The drawing under review shows one solid part. Ordinate dimensions are in mm from its lowest x, y, z. A direction names the side the tool comes from. Coordinates: 2 decimals unless noted, no trailing zeros. Order: outer loops, then holes, each group sorted by start corner. A loop starts at its lowest first (then second) coordinate and runs counter-clockwise, first axis right, second up.
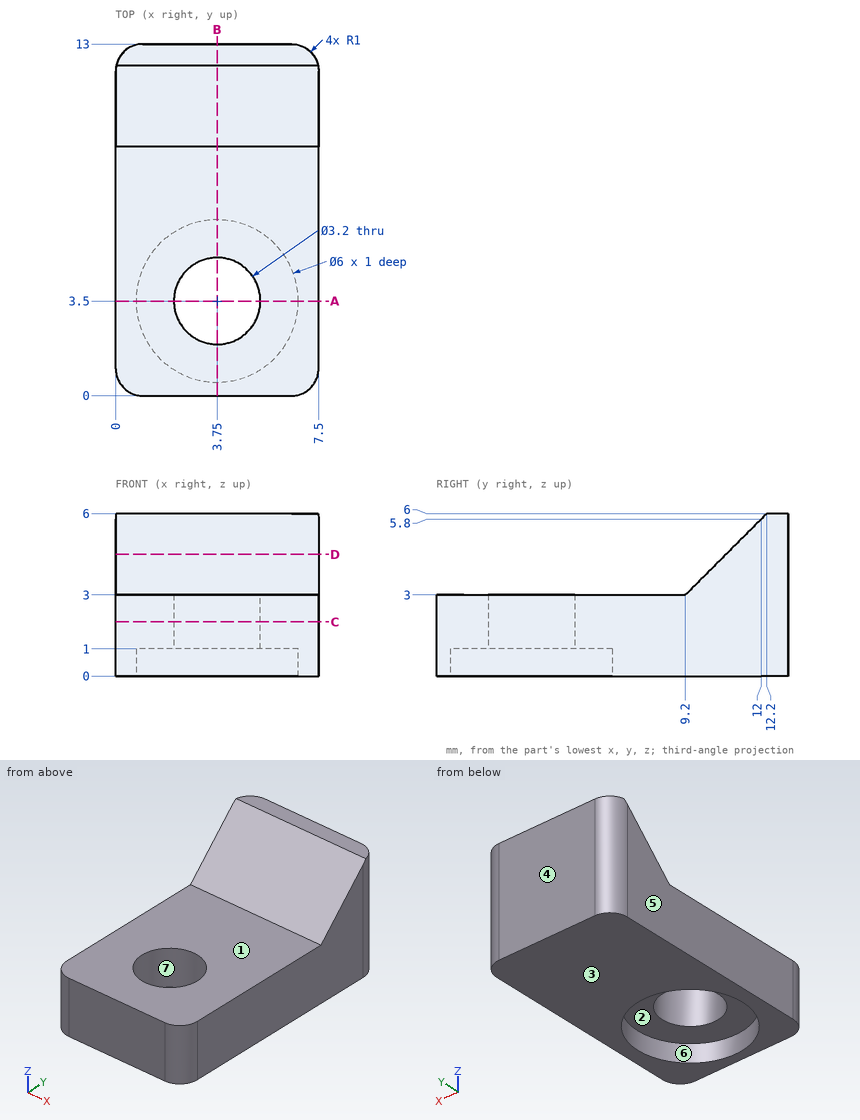
1. Take a section at D-D, the plane z = 4.5. Give the boundary of the cut face in (x, y), plus the area to 3 significant figures.
Answer below:
outline: (0, 10.7) - (7.5, 10.7) - (7.5, 12) arc R1 ccw to (6.5, 13) - (1, 13) arc R1 ccw to (0, 12) - close
area: 16.8 mm2
2. Take a section at C-C, the plane z = 2. Give the boundary of the cut face in (x, y), plus the area to 3 significant figures.
Answer below:
outline: (0, 1) arc R1 ccw to (1, 0) - (6.5, 0) arc R1 ccw to (7.5, 1) - (7.5, 12) arc R1 ccw to (6.5, 13) - (1, 13) arc R1 ccw to (0, 12) - close; hole circle Ø3.2 at (3.75, 3.5)
area: 88.6 mm2
3. Take a section at A-A, the plane y = 3.5. Give the boundary of the cut face in (x, z), plus the area to 3 significant figures.
Answer below:
outline: (0, 0) - (0.75, 0) - (0.75, 1) - (2.15, 1) - (2.15, 3) - (0, 3) - close; (5.35, 1) - (6.75, 1) - (6.75, 0) - (7.5, 0) - (7.5, 3) - (5.35, 3) - close
area: 10.1 mm2
4. Machinability: for the marked faces 1, 2 and 3, which of the approach directions +Z, -Z, +X, -X, +Y, -Y give a long, thin tool a straight path to every point of the face, cutting with its end or side? Answer none if there is none.
Answer below:
face 1: +Z, +X, -X, -Y
face 2: -Z
face 3: -Z, +X, -X, +Y, -Y
5. The part is to be moulded in two halves that separate along X. For the marked faces 4, 5, 6 and 7, say which applies: +X half, -X half, draft (parallel to the pull), parting line (faces both ways), or undercut.
Answer below:
face 4: draft
face 5: -X half
face 6: undercut
face 7: undercut
6. To check wall thickness, follow L1, parallel to Y at x = 3.75, z = 2.2; L2, parallel to Y at x = 3.75, z = 0.6; L3, parallel to Z at x = 3, y = 8.5. State the ranges of each line that lie inside material, in increasing order.
Answer below:
L1: y = 0 to 1.9, 5.1 to 13
L2: y = 0 to 0.5, 6.5 to 13
L3: z = 0 to 3
7. Clearance check with flat-ended pins moving along their axes: pin 1 Ø1 at (x, y) = (6.5, 6) entering from -Z; pin 2 Ø2 at (x, y) = (3.5, 6) entering from +Z; pin 3 Ø3 at (x, y) = (6, 10) entering from +Z. State where each tip first meets the part, or that it passes through.
Answer below:
pin 1: stops at z = 0
pin 2: stops at z = 3
pin 3: stops at z = 5.3
8. Take a section at B-B, the plane x = 3.75. Give the boundary of the cut face in (y, z).
Answer below:
outline: (0, 0) - (0.5, 0) - (0.5, 1) - (1.9, 1) - (1.9, 3) - (0, 3) - close; (5.1, 1) - (6.5, 1) - (6.5, 0) - (13, 0) - (13, 6) - (12.2, 6) - (9.2, 3) - (5.1, 3) - close
